```python
from build123d import *

# Parameters (mm, degrees)
SKETCH1_W           = 38.1
SKETCH1_H           = 43.18
BOSS_EXTRUDE1_DEPTH = 2.54
SKETCH2_W           = 29.845
SKETCH2_H           = 35.56
BOSS_EXTRUDE2_DEPTH = 2.54
SKETCH3_W           = 25.4
SKETCH3_H           = 35.56
BOSS_EXTRUDE3_DEPTH = 4
SKETCH7_W           = 20.32
SKETCH7_H           = 3.81
BOSS_EXTRUDE5_DEPTH = 6.54
FILLET1_R           = 1.905


with BuildPart() as part:
    # Sketch1 → Boss-Extrude1 (new body)
    with BuildSketch(Plane(origin=(0, 0, 0), x_dir=(1, 0, 0), z_dir=(0, 1, 0))):
        with Locations((-0.216477273, -10.297102273)):
            Rectangle(SKETCH1_W, SKETCH1_H)
    extrude(amount=BOSS_EXTRUDE1_DEPTH)

    # Sketch2 → Boss-Extrude2 (add)
    with BuildSketch(Plane(origin=(0, 2.54, 0), x_dir=(1, 0, 0), z_dir=(0, 1, 0))):
        with Locations((-0.216477273, -10.297102273)):
            Rectangle(SKETCH2_W, SKETCH2_H)
    extrude(amount=BOSS_EXTRUDE2_DEPTH)

    # Sketch3 → Boss-Extrude3 (add)
    with BuildSketch(Plane(origin=(0, 5.08, 0), x_dir=(1, 0, 0), z_dir=(0, 1, 0))):
        with Locations((-0.406977273, -10.297102273)):
            Rectangle(SKETCH3_W, SKETCH3_H)
    extrude(amount=BOSS_EXTRUDE3_DEPTH)

    # Sketch7 → Boss-Extrude5 (add)
    with BuildSketch(Plane(origin=(0, 2.54, 0), x_dir=(1, 0, 0), z_dir=(0, 1, 0))):
        with Locations((-0.216477273, -29.982102273)):
            Rectangle(SKETCH7_W, SKETCH7_H)
        with Locations((-0.216477273, 9.387897727)):
            Rectangle(SKETCH7_W, SKETCH7_H)
    extrude(amount=BOSS_EXTRUDE5_DEPTH)

    # Fillet1
    fillet1_edges = [part.edges().sort_by_distance(p)[0] for p in [
        (-0.216477273, 0, -11.292897727),
        (18.833522727, 0, 10.297102273),
        (-0.216477273, 0, 31.887102273),
        (-19.266477273, 0, 10.297102273),
    ]]
    fillet(fillet1_edges, radius=FILLET1_R)


solid = part.part
```
Can you work these out from the model? Positions are in its coordinate system, mm. A direction names the side the tool comes from. Round coordinates to 2 decimals unless told otherwise and drop trailing zeros. Loops run counter-clockwise (first coordinate to the right, second up) from the corner with the lowest first, then second, coordinate; pieces in that order, holes last. Notation, with made-up numbers: M -20.75,-16.75 L 32.25,-16.75 A18 ccw 32.25,14.25 Z; hole C -2.75,25 d4. An arc over 180 degrees is marked long. Write item = value, one per line. Start each with the question number.
(1) Suppose I cut it at B-B on z = -2.5. Write out the boundary of the cut face in (x, y) (3 decimals), plus the area to 3 significant figures.
(2) Suppose I cut it at C-C on y = 7.5. Write out the boundary of the cut face in (x, z), plus the area to 3 significant figures.
(3) Suppose I cut it at A-A on y = 4. Write out the boundary of the cut face in (x, z), plus the area to 3 significant figures.
(4) Which directions (+Z, -Z, +X, -X, +Y, -Y) give clear straight access to the entire face, cutting with the end or side of a thin tool? Please do faces 1 (the face through (13, 5.08, 10)), 2 (the face through (12, 5, -7.483)), 3 (the face through (9.944, 6, 30)).
(5) I'm going to push flat-ended pins straight in: P1, Ø2, axis at y = 7, z = 16.5, coming from the -X side; P2, Ø1.4, axis at x = 12, y = 7, coming from the -Z side; P3, Ø1, axis at x = -14, z = 14.5, coming from the +Y side. Where does each tip first touch, or does it pass through?
(6) I need wall thicknesses on line 1 along Y through (x, z) = (-15.5, 24); line 2 along X through (y, z) = (5.25, -9); line 3 along Y through (x, z) = (14, 3). Which ranges of each line are inside material? Lowest first, please.
Answer block:
q1.outline = M -19.266,1.905 A1.905 ccw -17.361,0 L 16.929,0 A1.905 ccw 18.834,1.905 L 18.834,2.54 L 14.706,2.54 L 14.706,5.08 L 12.293,5.08 L 12.293,9.08 L -13.107,9.08 L -13.107,5.08 L -15.139,5.08 L -15.139,2.54 L -19.266,2.54 Z
q1.area = 273 mm²
q2.outline = M -13.11,-7.48 L -10.38,-7.48 L -10.38,-11.29 L 9.94,-11.29 L 9.94,-7.48 L 12.29,-7.48 L 12.29,28.08 L 9.94,28.08 L 9.94,31.89 L -10.38,31.89 L -10.38,28.08 L -13.11,28.08 Z
q2.area = 1,060 mm²
q3.outline = M -15.14,-7.48 L -10.38,-7.48 L -10.38,-11.29 L 9.94,-11.29 L 9.94,-7.48 L 14.71,-7.48 L 14.71,28.08 L 9.94,28.08 L 9.94,31.89 L -10.38,31.89 L -10.38,28.08 L -15.14,28.08 Z
q3.area = 1,220 mm²
q4.face_1 = +Z, -Z, +X, +Y
q4.face_2 = -Z, +X, +Y
q4.face_3 = +Z, +X, +Y
q5.P1 = -13.11
q5.P2 = -7.48
q5.P3 = 5.08
q6.line_1 = 0 to 2.54
q6.line_2 = -10.38 to 9.94
q6.line_3 = 0 to 5.08
